from build123d import *

# Parameters (mm, degrees)
SKETCH1_W            = 50
SKETCH1_H            = 50
BOSS_EXTRUDE1_DEPTH  = 2
SKETCH2_W            = 8.5
SKETCH2_H            = 2
SKETCH2_W_2          = 25.5
BOSS_EXTRUDE2_DEPTH  = 20
SKETCH3_W            = 2
SKETCH3_H            = 15
BOSS_EXTRUDE3_DEPTH  = 20
SKETCH5_W            = 2
SKETCH5_H            = 15
BOSS_EXTRUDE5_DEPTH  = 25
SKETCH8_W            = 3.5
SKETCH8_H            = 6
BOSS_EXTRUDE7_DEPTH  = 8
BOSS_EXTRUDE8_DEPTH  = 3.5
SKETCH10_W           = 9
SKETCH10_H           = 9
SKETCH10_R           = 1.5
SKETCH10_R_2         = 1.65
SKETCH10_W_2         = 10
SKETCH10_H_2         = 10
BOSS_EXTRUDE9_DEPTH  = 2
FILLET1_R            = 5
SKETCH11_W           = 17
SKETCH11_H           = 3
BOSS_EXTRUDE10_DEPTH = 19
FILLET2_R            = 1.5
SKETCH12_W           = 13
SKETCH12_H           = 10
BOSS_EXTRUDE11_DEPTH = 4
FILLET3_START        = -2
FILLET3_DEPTH        = 4
FILLET3_START_2      = -20
FILLET3_2_DEPTH      = 18.41096
FILLET3_3_DEPTH      = 2
SKETCH13_R           = 1.425
CUT_EXTRUDE1_DEPTH   = 105.091306073
FILLET4_START        = -2.000000956
FILLET4_DEPTH        = 4.000000956
FILLET4_START_2      = -30
FILLET4_2_DEPTH      = 5


with BuildPart() as part:
    # Sketch1 → Boss-Extrude1 (new body)
    with BuildSketch(Plane.XY):
        Rectangle(SKETCH1_W, SKETCH1_H)
    extrude(amount=BOSS_EXTRUDE1_DEPTH)

    # Sketch2 → Boss-Extrude2 (add)
    with BuildSketch(Plane(origin=(0, 0, 0), x_dir=(-1, 0, 0), z_dir=(0, 0, -1))):
        with Locations((-20.75, -24)):
            Rectangle(SKETCH2_W, SKETCH2_H)
        with Locations((12.25, -24)):
            Rectangle(SKETCH2_W_2, SKETCH2_H)
    extrude(amount=BOSS_EXTRUDE2_DEPTH)

    # Sketch3 → Boss-Extrude3 (add)
    with BuildSketch(Plane.XZ.offset(25)):
        with Locations((24, -5.5)):
            Rectangle(SKETCH3_W, SKETCH3_H)
    extrude(amount=BOSS_EXTRUDE3_DEPTH)

    # Sketch5 → Boss-Extrude5 (add)
    with BuildSketch(Plane(origin=(0, 0, 0), x_dir=(-1, 0, 0), z_dir=(0, 0, -1))):
        with Locations((-20.5, 5.5)):
            Rectangle(SKETCH5_W, SKETCH5_H)
        with Locations((22, 5.5)):
            Rectangle(SKETCH5_W, SKETCH5_H)
    extrude(amount=BOSS_EXTRUDE5_DEPTH)

    # Sketch8 → Boss-Extrude7 (add)
    with BuildSketch(Plane(origin=(0, 0, 0), x_dir=(-1, 0, 0), z_dir=(0, 0, -1))):
        with Locations((23.25, -11)):
            Rectangle(SKETCH8_W, SKETCH8_H)
    extrude(amount=BOSS_EXTRUDE7_DEPTH)

    # Sketch9 → Boss-Extrude8 (add)
    with BuildSketch(Plane(origin=(25, 0, 0), x_dir=(0, 0, -1), z_dir=(1, 0, 0))):
        Polygon((-2, 25), (0, 25), (0, -23), (20, -23), (20, -25), (13, -25), (13, -45), (-2, -45), align=None)
    extrude(amount=BOSS_EXTRUDE8_DEPTH)

    # Mirror1: part across plane


with BuildPart() as part_1:
    add(part.part)
    add(part.part.mirror(Plane.ZY.offset(-28.5)))

    # Sketch10 → Boss-Extrude9 (add)
    # profile 1 of 3: a face of its own
    with BuildSketch(Plane(origin=(0, 0, 0), x_dir=(-1, 0, 0), z_dir=(0, 0, -1))):
        with Locations((-86.5, -9)):
            Rectangle(SKETCH10_W, SKETCH10_H)
        with Locations((-88.5, -9)):
            Circle(SKETCH10_R, mode=Mode.SUBTRACT)
    # profile 2 of 3: a face of its own
    with BuildSketch(Plane(origin=(0, 0, 0), x_dir=(-1, 0, 0), z_dir=(0, 0, -1))):
        Polygon((-79.85, 35), (-79.85, 25), (-82, 25), (-82, 22.35), (-91, 22.35), (-91, 35), align=None)
        with Locations((-88.5, 31)):
            Circle(SKETCH10_R_2, mode=Mode.SUBTRACT)
    # profile 3 of 3: a face of its own
    with BuildSketch(Plane(origin=(0, 0, 0), x_dir=(-1, 0, 0), z_dir=(0, 0, -1))):
        with Locations((-48.5, 30)):
            Rectangle(SKETCH10_W_2, SKETCH10_H_2)
        with Locations((-48.5, 31)):
            Circle(SKETCH10_R, mode=Mode.SUBTRACT)
    extrude(amount=-BOSS_EXTRUDE9_DEPTH)

    # Fillet1
    # the kernel refuses this fillet: 5 mm, written as the material it adds along each edge
    with BuildSketch(Plane(origin=(82, -4.5, 0), x_dir=(0, 1, 0), z_dir=(0, 0, 1)), Plane(origin=(79.85, 25, 0), x_dir=(-1, 0, 0), z_dir=(0, 0, 1)), Plane(origin=(43.5, 25, 0), x_dir=(-1, 0, 0), z_dir=(0, 0, 1))) as fillet1_piece_1:
        with BuildLine():
            CenterArc((FILLET1_R, -FILLET1_R), FILLET1_R, 90, 90)
            Line((0, -FILLET1_R), (0, 0))
            Line((0, 0), (FILLET1_R, 0))
        make_face()
    extrude(amount=2)
    with BuildSketch(Plane(origin=(82, -13.5, 0), x_dir=(0, -1, 0), z_dir=(0, 0, 1)), Plane(origin=(82, 22.35, 0), x_dir=(0, -1, 0), z_dir=(0, 0, 1)), Plane(origin=(53.5, 25, 0), x_dir=(1, 0, 0), z_dir=(0, 0, 1))) as fillet1_piece_2:
        with BuildLine():
            CenterArc((FILLET1_R, FILLET1_R), FILLET1_R, 180, 90)
            Line((0, FILLET1_R), (0, 0))
            Line((0, 0), (FILLET1_R, 0))
        make_face()
    extrude(amount=2)

    # Sketch11 → Boss-Extrude10 (add)
    with BuildSketch(Plane(origin=(0, 0, 0), x_dir=(-1, 0, 0), z_dir=(0, 0, -1))):
        with Locations((-70.2, -17.4)):
            Rectangle(SKETCH11_W, SKETCH11_H)
        with Locations((12.5, -17.4)):
            Rectangle(SKETCH11_W, SKETCH11_H)
    extrude(amount=BOSS_EXTRUDE10_DEPTH)

    # Fillet2
    fillet2_edges = [part_1.edges().sort_by_distance(p)[0] for p in [
        (79, 13, 0),
        (79, -2, 0),
        (80, 5.5, 0),
        (36.5, 13, 0),
        (35.5, 5.5, 0),
        (36.5, -2, 0),
        (20.5, 13, 0),
        (20.5, -2, 0),
        (21.5, 5.5, 0),
        (-22, 13, 0),
        (-23, 5.5, 0),
        (-22, -2, 0),
    ]]
    fillet(fillet2_edges, radius=FILLET2_R)

    # Sketch12 → Boss-Extrude11 (add)
    with BuildSketch(Plane.XY.offset(2)):
        with Locations((-31.5, -16.5)):
            Rectangle(SKETCH12_W, SKETCH12_H)
    extrude(amount=-BOSS_EXTRUDE11_DEPTH)

    # Fillet3: read off the stored shape, not the designer's step
    # Fillet3 outline → Fillet3 (add)
    with BuildSketch(Plane.XY.offset(FILLET3_START)):
        with BuildLine():
            ThreePointArc((-25.846127967, -23), (-25.284740857, -23.941480467), (-25, -25))
            Line((-25, -25), (-25, -23))
            Line((-25, -23), (-25.846127967, -23))
        make_face()
        with BuildLine():
            ThreePointArc((-25.031373033, -8), (-26.354248689, -10.5), (-29, -11.5))
            Line((-29, -11.5), (-25, -11.5))
            Line((-25, -11.5), (-25, -8))
            Line((-25, -8), (-25.031373033, -8))
        make_face()
    extrude(amount=FILLET3_DEPTH)

    # Fillet3 2 outline → Fillet3 2 (add)
    with BuildSketch(Plane.XY.offset(FILLET3_START_2)):
        with BuildLine():
            ThreePointArc((-25.846127967, -23), (-25.284740857, -23.941480467), (-25, -25))
            Line((-25, -25), (-25, -23))
            Line((-25, -23), (-25.846127967, -23))
        make_face()
    extrude(amount=FILLET3_2_DEPTH)

    # Fillet3 3 outline → Fillet3 3 (add)
    with BuildSketch(Plane.XY):
        with BuildLine():
            ThreePointArc((-28.968626967, -21.5), (-27.236576159, -21.894448725), (-25.846127967, -23))
            Line((-25.846127967, -23), (-25, -23))
            Line((-25, -23), (-25, -21.5))
            Line((-25, -21.5), (-28.968626967, -21.5))
        make_face()
        with BuildLine():
            ThreePointArc((-25, -7.5), (-25.007850963, -7.75049165), (-25.031373033, -8))
            Line((-25.031373033, -8), (-25, -8))
            Line((-25, -8), (-25, -7.5))
        make_face()
    extrude(amount=FILLET3_3_DEPTH)

    # Sketch13 → Cut-Extrude1 (cut, through all)
    with BuildSketch(Plane(origin=(0, 0, -2), x_dir=(-1, 0, 0), z_dir=(0, 0, -1))):
        with Locations((33, -16.5)):
            Circle(SKETCH13_R)
    extrude(amount=-CUT_EXTRUDE1_DEPTH, mode=Mode.SUBTRACT)

    # Fillet4: read off the stored shape, not the designer's step
    # Fillet4 outline → Fillet4 (add)
    with BuildSketch(Plane.XY.offset(FILLET4_START)):
        with BuildLine():
            Line((-25.846127967, -23), (-25, -23))
            Line((-25, -23), (-25, -21.5))
            Line((-25, -21.5), (-28.968626967, -21.5))
            ThreePointArc((-28.968626967, -21.5), (-27.236576159, -21.894448725), (-25.846127967, -23))
        make_face()
    extrude(amount=FILLET4_DEPTH)

    # Fillet4 2 outline → Fillet4 2 (cut)
    with BuildSketch(Plane.YZ.offset(FILLET4_START_2)):
        with BuildLine():
            ThreePointArc((-21.499991299, -2.000015071), (-22.150318116, -1.157004674), (-23, -0.515418986))
            Line((-23, -0.515418986), (-23, -2.000000956))
            Line((-23, -2.000000956), (-21.499991299, -2.000015071))
        make_face()
    extrude(amount=FILLET4_2_DEPTH, mode=Mode.SUBTRACT)


solid = part_1.part
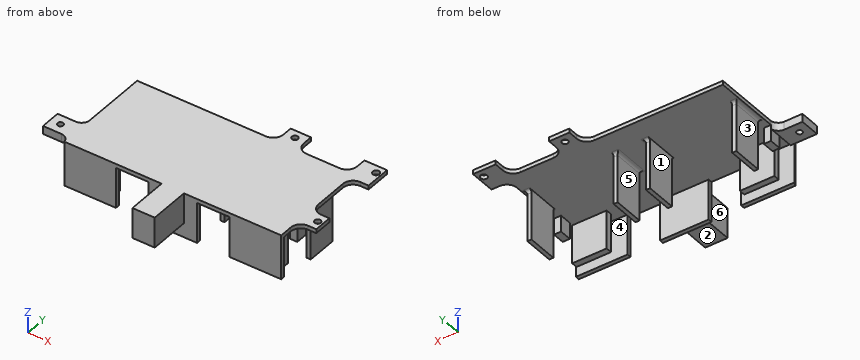
Model file for the job. Use its own axes, mm. Face numbers are marked on the shaded views. A direction names the side the tool comes from. Coordinates: 2 decimals unless noted, no trailing zeros. Write each loop counter-clockwise with the first axis right and the second up, starting at its lowest first coordinate (ties: lowest second). Pieces come first, ordered by that corner, then holes. Notation, with made-up numbers: (-14.5, 13.25) -> (13.5, 13.25) arc R28 cw to (13.5, 45.25) -> close; hole circle Ø1 at (-15, 42). An arc over 180 degrees is marked (long way). One line per item, written item: value. Start each with the question number.
1) Slice it at B-B on x = -13.5. Write the cut outline in (y, z).
2) Pull direction X, two halves, no side cores. Call the marked faces 4, 5 and 6: +X half, -X half, draft (parallel to the pull), parting line (faces both ways), or undercut.
3) Slice it at A-A on x = -33. Write the cut outline in (y, z) (3 decimals).
4) Flat gauge pins, fed straight in: pin 1 Ø3 at (x, y) = (-12.5, 23.5) entering from -Z; pin 2 Ø1 at (y, z) = (9, -21) entering from -X; pin 3 Ø1 at (x, y) = (-8, -24) entering from -Z; pin 4 Ø6.5 at (y, z) = (-11.5, -3.5) entering from -X. Where does each tip first touch, or does it go through?
5) Which spindle directions (+Z, -Z, +X, -X, +Y, -Y) get a long thin tool onto all of the face, cutting with end or side? Do the marked faces 1, 2 and 3. Say none if no direction does.
6) Probe probe 1 along X at (y, z) = (-1.5, -4); probe 2 along Y at (x, z) = (-11, -0.75); probe 3 along Y at (x, z) = (48.5, 0.7). List the from-to ranges inside material, lowest first.
7) Slice it at C-C on z = -3.75. Count the separate pieces of the cut face and the enclosed holes in it, then the cut area to 3 significant figures.
8) Slice it at D-D on x = 48.5. Write the cut outline in (y, z), then the cut area to 3 significant figures.
Answers follow:
1. outline: (-25, -20) -> (-23, -20) -> (-23, 0) -> (-18.9, 0) -> (-18.9, -19) -> (-15.9, -19) -> (-15.9, 0) -> (25, 0) -> (25, 2) -> (-25, 2) -> close
2. face 4: draft
2. face 5: undercut
2. face 6: -X half
3. outline: (-21.5, -2) -> (-17.925, -2) -> (-17.925, 2) -> (-21.5, 2) -> close; (-15.075, -2) -> (-11.5, -2) -> (-11.5, 2) -> (-15.075, 2) -> close
4. pin 1: z = 0
4. pin 2: x = -23
4. pin 3: z = -20
4. pin 4: x = -38
5. face 1: -Z, +Y
5. face 2: -Z, +X, -X, -Y
5. face 3: -Z, -X, +Y
6. probe 1: -23 to -21, 19.5 to 21.5, 35.5 to 37.5, 78 to 80
6. probe 2: -25 to -23, -18.9 to -15.9
6. probe 3: -25 to 29.5, 32.5 to 35
7. separate pieces: 11
7. enclosed holes: 0
7. area: 635 mm2
8. outline: (-25, 0) -> (29.5, 0) -> (29.5, 2) -> (-25, 2) -> close; (32.5, 0) -> (35, 0) -> (35, 2) -> (32.5, 2) -> close
8. area: 114 mm2
